from build123d import *

# Parameters (mm, degrees)
ESQUISSE1_R             = 3.5
BOSS_EXTRU_1_DEPTH      = 4
ESQUISSE2_R             = 2
BOSS_EXTRU_2_DEPTH      = 25
ENL_V_MAT_EXTRU_1_DEPTH = 3
CHANFREIN1_SIZE         = 0.5
CONG_1_R                = 0.5


with BuildPart() as part:
    # Esquisse1 → Boss.-Extru.1 (new body)
    with BuildSketch(Plane.XY):
        Circle(ESQUISSE1_R)
    extrude(amount=BOSS_EXTRU_1_DEPTH)

    # Esquisse2 → Boss.-Extru.2 (add)
    with BuildSketch(Plane.XY.offset(4)):
        Circle(ESQUISSE2_R)
    extrude(amount=BOSS_EXTRU_2_DEPTH)

    # Esquisse3 → Enlèv. mat.-Extru.1 (cut)
    with BuildSketch(Plane(origin=(0, 0, 0), x_dir=(-1, 0, 0), z_dir=(0, 0, -1))):
        Polygon((1.732050808, 0), (0.866025404, 1.5), (-0.866025404, 1.5), (-1.732050808, 0), (-0.866025404, -1.5), (0.866025404, -1.5), align=None)
    extrude(amount=-ENL_V_MAT_EXTRU_1_DEPTH, mode=Mode.SUBTRACT)

    # Chanfrein1
    chanfrein1_edges = [part.edges().sort_by_distance(p)[0] for p in [
        (-2, 0, 29),
    ]]
    chamfer(chanfrein1_edges, length=CHANFREIN1_SIZE)

    # Congé1
    cong_1_edges = [part.edges().sort_by_distance(p)[0] for p in [
        (-3.5, 0, 0),
    ]]
    fillet(cong_1_edges, radius=CONG_1_R)


solid = part.part
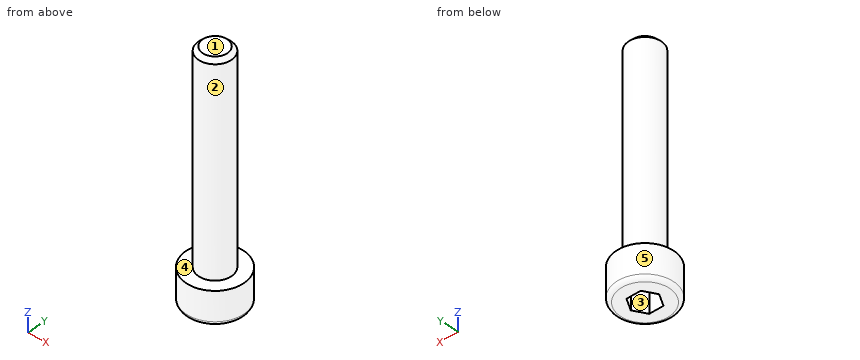
The model under review builds one solid part; all positions refer to its coordinate system, in mm. Face numbers are marked on the shaded views. A direction names the side the tool comes from. Round coordinates to 2 decimals unless told otherwise and drop trailing zeros. Write each loop counter-clockwise with the first axis right and the second up, starting at its lowest first coordinate (ties: lowest second). Pieces come first, ordered by that corner, then holes. Notation, with made-up numbers: M 57.5,88 L 68.5,88 A11 cw 68.5,108 Z; hole C 40.5,17 d11. An arc over 180 degrees is marked long. Answer as CSV lines item,"result". Start each with the question number.
Q1. Tool access review of the marked faces 1 and 2: name each direction out of +Z, -Z, +X, -X, +Y, -Y from which nothing blocks a thin tool from reaching the whole face with its end or side.
Q2. Consider section B-B, the plane z = 16. Give the boundary of the cut face in (x, y).
Q3. Consider section A-A, the plane x = 0. Give the boundary of the cut face in (y, z).
Q4. Wall thickness on line 1 along Z through (x, y) = (-2.25, -2); line 2 along Y through (x, z) = (-1, 16); line 3 along Z through (x, y) = (1.25, 0.75): over which ranges is each line inside the solid? List them lowest first.
Q5. The part is to be moulded in two halves that separate along Y. For the marked faces 3, 4 and 5, say which applies: +Y half, -Y half, draft (parallel to the pull), parting line (faces both ways), or undercut.
Q6. Clearance check with flat-ended pins moving along their axes: P1, Ø2, axis at x = -2, y = 0.5, coming from the +Z side; P2, Ø1, axis at y = -1, z = 5, coming from the +X side; P3, Ø1.5, axis at x = 0.5, y = 0.5, coming from the -Z side; P4, Ø1, axis at y = -2, z = 19.5, coming from the -X side. State where each tip first meets the part, or that it passes through.
Result set:
1,face 1,"+Z, +X, -X, +Y, -Y"
1,face 2,"+Z"
2,outline,"C 0,0 d4"
3,outline,"M -3.5,0.5 A0.5 ccw -3,0 L -1.5,0 L -1.5,3 L 1.5,3 L 1.5,0 L 3,0 A0.5 ccw 3.5,0.5 L 3.5,4 L 2,4 L 2,28.5 L 1.5,29 L -1.5,29 L -2,28.5 L -2,4 L -3.5,4 Z"
4,line 1,"z = 0 to 4"
4,line 2,"y = -1.73 to 1.73"
4,line 3,"z = 3 to 29"
5,face 3,"undercut"
5,face 4,"draft"
5,face 5,"parting line"
6,P1,"stops at z = 29"
6,P2,"stops at x = 1.94"
6,P3,"stops at z = 3"
6,P4,"stops at x = -1.32"
